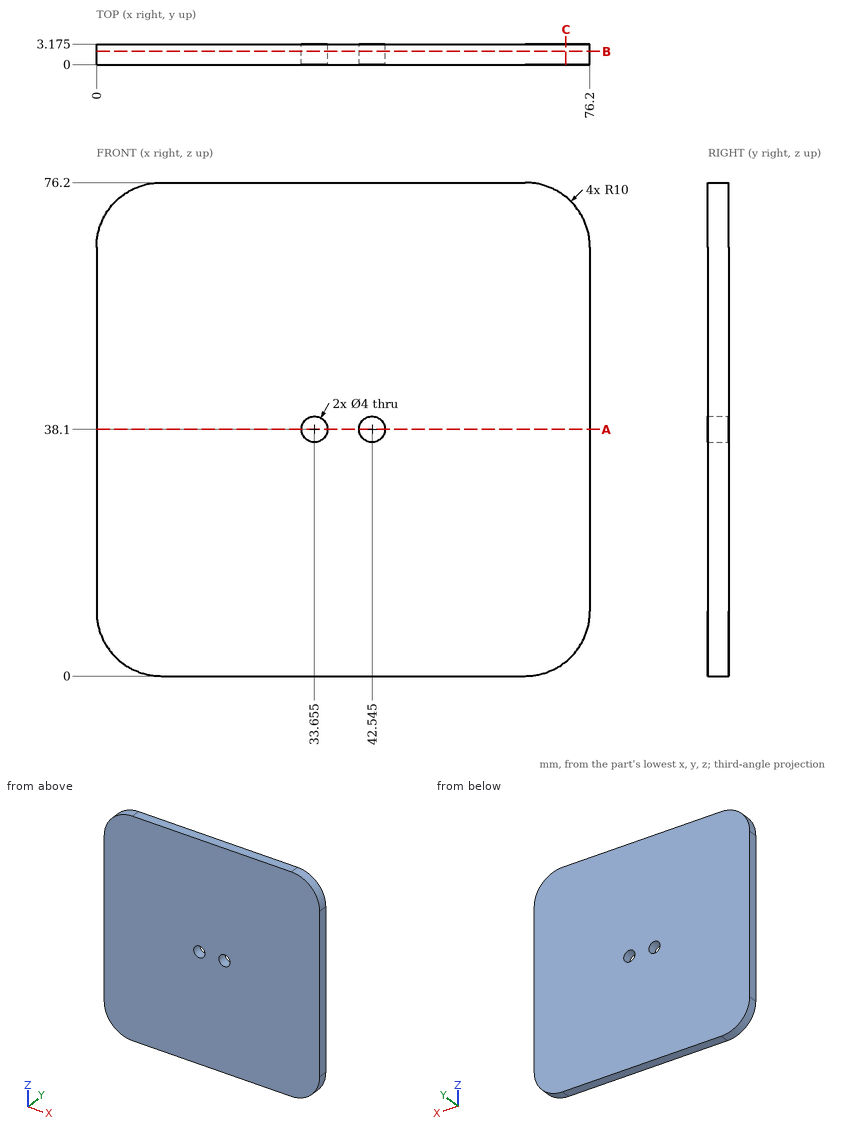
Design review of the part shown in the three views and the two pictorial views. Dimensions are in mm from the part's minimum x, y and z. Coordinates: 2 decimals unless noted, no trailing zeros. Order: outer loops, then holes, each group sorted by start corner. A loop starts at its lowest first (then second) coordinate and runs counter-clockwise, first axis right, second up. Notation, with made-up numbers: (58.5, -15.5) - (79.5, -15.5) arc R19 ccw to (79.5, -3.5) - close; hole circle Ø5 at (-37, -7.75). An arc over 180 degrees is marked (long way). Answer as CSV lines item,"result". Start each with the question number.
1) To check wall thickness, follow line 1 along X through (y, z) = (1.6, 38.1) (3 decimals); line 2 along X through (y, z) = (1.3, 36.5) (3 decimals); line 3 along Z through (x, y) = (8, 0.25). State the ranges of each line that lie inside material, in increasing order. Write a range as [from, to].
2) Add section C-C (x = 72.5). State the section outline as (y, z) points (3 decimals), then the cut area to 3 significant figures.
3) Add section A-A (z = 38.1). State the section outline as (x, y) points (3 decimals).
4) Add section B-B (y = 2.05). State the section outline as (x, z) points (3 decimals), then the cut area to 3 significant figures.
Result:
1,line 1,"[0, 31.655], [35.655, 40.545], [44.545, 76.2]"
1,line 2,"[0, 32.455], [34.855, 41.345], [43.745, 76.2]"
1,line 3,"[0.2, 76]"
2,outline,"(0, 2.234) - (3.175, 2.234) - (3.175, 73.966) - (0, 73.966) - close"
2,area,"228 mm^2"
3,outline,"(0, 0) - (31.655, 0) - (31.655, 3.175) - (0, 3.175) - close; (35.655, 0) - (40.545, 0) - (40.545, 3.175) - (35.655, 3.175) - close; (44.545, 0) - (76.2, 0) - (76.2, 3.175) - (44.545, 3.175) - close"
4,outline,"(0, 10) arc R10 ccw to (10, 0) - (66.2, 0) arc R10 ccw to (76.2, 10) - (76.2, 66.2) arc R10 ccw to (66.2, 76.2) - (10, 76.2) arc R10 ccw to (0, 66.2) - close; hole circle Ø4 at (33.655, 38.1); hole circle Ø4 at (42.545, 38.1)"
4,area,"5,700 mm^2"
